Build history of the part. All positions in model axes, mm. A direction names the side the tool comes from. Coordinates: 2 decimals unless noted, no trailing zeros. Order: outer loops, then holes, each group sorted by start corner. A loop starts at its lowest first (then second) coordinate and runs counter-clockwise, first axis right, second up. Notation, with made-up numbers: M 72.25,11.25 L 100.25,11.25 A20 ccw 100.25,17.25 Z; hole C -36,-16 d2. An arc over 180 degrees is marked long. Write item = value, one per line. Start each with the question number.
Q1. 3-axis set-ups, long thin cutter, end or side, ignore diameter. For faces 4 (the face through (-19, 3.175, -19)), 5 (the face through (-60.456, 18.158, 0.269)): which of +Z, -Z, +X, -X, +Y, -Y reach the whole face in a straight line?
Q2. Pin check, flat tips, straight feed: P1, Ø5, axis at y = 37, z = -19.5, coming from the -X side; P2, Ø7.5, axis at x = -26.543, z = 0, coming from the +Y side (3 decimals); P3, Ø4, axis at x = 0, z = -26.543, coming from the +Y side; P4, Ø4, axis at x = -43.5, y = 21.5, coming from the -Z side. Stop position of each tip, or through.
Q3. Band-saw the part on A-A on y = 18. Write the cut outline in (x, z).
Q4. Band-saw the part on C-C on y = 27.5. Write the cut outline in (x, z).
Q5. Drill centre lines: probe 1 along Y at (x, z) = (-13, -11) (3 decimals); probe 2 along X at (y, z) = (35.5, -13.5); probe 3 along Z at (x, y) = (-2.5, 27). Where is each one in solid material? Low to high.
Q6. Band-saw the part on B-B on z = -57.5. State how many separate pieces and enclosed holes the cut face has, plus the area to 3 significant figures.
Q7. Pull direction Y, two halves, no side cores. Call faces 1 (the face through (-3.253, 37.208, -56.935)), 2 (the face through (-1.5, 1.6, -23.6)), 3 (the face through (-31, 44.45, -30)): released by +Y, released by -Y, zero draft, split by the parting line, or undercut.
Autodesk Inventor part; units mm, degrees
ref_plane "YZ Plane" through (0, 0, 0) normal (1, 0, 0) x (0, 1, 0)
ref_plane "XZ Plane" through (0, 0, 0) normal (0, 1, 0) x (-1, 0, 0)
ref_plane "XY Plane" through (0, 0, 0) normal (0, 0, 1) x (1, 0, 0)
sketch "Sketch1" plane through (0, 0, 0) normal (0, 1, 0) x (-1, 0, 0)
  circle A0 centre (0, 0) radius 26.543 construction
  circle A1 centre (0, 26.543) radius 3.302
  circle A2 centre (26.543, 0) radius 3.302
  circle A3 centre (0, -26.543) radius 3.302
  circle A4 centre (-26.543, 0) radius 3.302
  circle A5 centre (0, 0) radius 12.7
  line L0 (0, 0) -> (-8.4134, 0) construction
  line L1 (10.9985, 6.35) -> (59.8338, 6.35)
  line L2 (-6.35, -10.9985) -> (-6.35, -59.8338)
  line L3 (59.8338, 6.35) -> (-6.35, -59.8338)
  dimension "d0" = 53.086
  dimension "d1" = 6.604
  dimension "d2" = 6.604
  dimension "d3" = 6.604
  dimension "d4" = 6.604
  dimension "d5" = 25.4
  dimension "d8" = 6.35
  dimension "d9" = 0
  dimension "d10" = 6.35
  dimension "d11" = 6.35
  dimension "d12" = 45
  dimension "d13" = 19.05
extrude "Plate1" add sketch "Sketch1" along normal blind 3.175 contours A5 L1 L3 L2
sketch "Sketch2" plane through (-62.0788, 6.35, 4.1049) normal (-0.7071068, 0, -0.7071068) x (0, -1, 0)
  line L0 (0, -93.598) -> (0, 0)
  line L1 (0, 0) -> (-38.1, 0)
  line L2 (-38.1, 0) -> (-38.1, -93.598)
  line L3 (-38.1, -93.598) -> (0, -93.598)
edge flange "Flange1" height 44.45 angle 90 thickness 3.175 bend radius 3.175 thickness toward (-0.7071068, 0, -0.7071068) relief tear relief width 3.175 relief depth 1.5875 edges at (-26.7419, 3.175, -26.7419) wall of the first edge with corners at (4.1049, 6.35, -62.0788) (-62.0788, 6.35, 4.1049) (-62.0788, 44.45, 4.1049) (4.1049, 44.45, -62.0788)
bend "Bend1"
corner "Corner1"
sketch "Sketch3" plane through (4.1049, 6.35, -62.0788) normal (0.7071068, 0, 0.7071068) x (0.7071068, 0, -0.7071068)
  line L0 (0, 38.1) -> (-93.598, 38.1)
  line L1 (0, 38.1) -> (0, 0)
  line L2 (-93.598, 38.1) -> (-93.598, 0)
  line L3 (-93.598, 0) -> (0, 0)
  circle A0 centre (-87.248, 28.575) radius 3.3782
  circle A1 centre (-6.35, 28.575) radius 3.3782
  circle A2 centre (-6.35, 9.525) radius 3.3782
  circle A3 centre (-87.248, 9.525) radius 3.3782
  point P0 (-46.799, -6.35)
  dimension "d35" = 93.598
  dimension "d36" = 6.7564
  dimension "d37" = 6.7564
  dimension "d38" = 6.7564
  dimension "d39" = 6.7564
  dimension "d40" = 6.35
  dimension "d41" = 9.525
  dimension "d42" = 9.525
  dimension "d43" = 6.35
  dimension "d44" = 9.525
  dimension "d45" = 9.525
  dimension "d47" = 6.35
  dimension "d48" = 6.35
extrude "Cut3" cut sketch "Sketch3" against normal blind 3.175 contours A0 | A1 | A2 | A3
equation "\"d49\" = Thickness"
equation "\"d15\" = BendReliefWidth"
equation "\"d16\" = BendReliefDepth"
equation "\"d17\" = MinimumRemnant"
equation "\"d18\" = BendRadius"
equation "\"d21\" = BendRadius"
equation "\"d22\" = CornerReliefSize"
equation "\"d23\" = GapSize"
equation "\"d24\" = JacobiRadiusSize"
equation "\"BendRadius\" = Thickness"
equation "\"BendReliefWidth\" = Thickness"
equation "\"BendReliefDepth\" = 0.5 * Thickness"
equation "\"CornerReliefSize\" = 4 * Thickness"
equation "\"MinimumRemnant\" = 2 * Thickness"
equation "\"TransitionRadius\" = BendRadius"
equation "\"JacobiRadiusSize\" = BendRadius"
equation "\"GapSize\" = Thickness"
equation "\"d14\" = BendRadius"
properties part number "Bearing Mount 3 v1" material "Aluminum 6061"
Recorded:
q1.face_4 = +Z, +X, +Y
q1.face_5 = none
q2.P1 = -45.46
q2.P2 = 3.175
q2.P3 = through
q2.P4 = -20.96
q3.outline = M -64.32,1.86 L -61.69,-0.77 L -59.45,1.47 L -62.08,4.1 Z; M -57.98,-4.49 L -4.49,-57.98 L -2.24,-55.73 L -55.73,-2.24 Z; M -0.77,-61.69 L 1.86,-64.32 L 4.1,-62.08 L 1.47,-59.45 Z
q4.outline = M -64.32,1.86 L 1.86,-64.32 L 4.1,-62.08 L -62.08,4.1 Z
q5.probe_1 = 0 to 3.175
q5.probe_2 = -48.96 to -44.47
q5.probe_3 = -59.96 to -55.47
q6.separate_pieces = 3
q6.enclosed_holes = 0
q6.area = 164 mm2
q7.face_1 = undercut
q7.face_2 = zero draft
q7.face_3 = released by +Y
